Read the model definition and answer for the solid it produces. Units are mm, in the model's axes. A direction names the side the tool comes from. Coordinates: 2 decimals unless noted, no trailing zeros. Write each loop counter-clockwise with the first axis right and the second up, starting at its lowest first coordinate (ties: lowest second). Pieces come first, ordered by that corner, then holes. Notation, with made-up numbers: (-27.75, -36) -> (25.25, -36) arc R31 ccw to (25.25, 1) -> close; hole circle Ø4 at (2, -20.5). An arc over 180 degrees is marked (long way). Return JSON: item names as keys, results as strings.
from build123d import *

# Parameters (mm, degrees)
F1_DEPTH = 50
F3_DEPTH = 50.001


with BuildPart() as f1:
    # F0 (on Front) → F1 (new body)
    with BuildSketch(Plane.XZ):
        Polygon((52.302633, -25), (52.302633, 25), (-47.697367, 25), (-77.697367, -25), (-47.697367, -25), (27.302633, -25), align=None)
        with BuildLine():
            ThreePointArc((-47.697367, -18.25), (-48.581251, -16.116117), (-46.447367, -17))
            ThreePointArc((-46.447367, -17), (-46.813484, -17.883883), (-47.697367, -18.25))
        make_face(mode=Mode.SUBTRACT)
        with BuildLine():
            ThreePointArc((27.302633, -18.25), (26.418749, -16.116117), (28.552633, -17))
            ThreePointArc((28.552633, -17), (28.186516, -17.883883), (27.302633, -18.25))
        make_face(mode=Mode.SUBTRACT)
    extrude(amount=F1_DEPTH)

    # F2 (on face) → F3 (cut, through all)
    with BuildSketch(Plane.XZ.offset(50)):
        Polygon((-47.697367, 25), (-62.697367, 0), (-28.942954, 0), (7.452939, 0), (52.302633, 15.462308), (52.302633, 25), align=None)
    extrude(amount=-F3_DEPTH, mode=Mode.SUBTRACT)


solid = f1.part
1. A tool of negligible diameter and unlimited length cuts with its end or side. For faces 4 (the face through (52.303, -25, -5)), 5 (the face through (-28, -25, 0)), from which of +Z, -Z, +X, -X, +Y, -Y can it reach the whole face along a straight path? Write none if from no direction.
Taken from the geometry:
{"face 4": "+Z, -Z, +X, +Y, -Y", "face 5": "+Z, -X, +Y, -Y"}
2. The part is cut by section A-A (y = -31.5). Determine the outline of the cut face in (x, z).
Taken from the geometry:
{"outline": "(-77.7, -25) -> (52.3, -25) -> (52.3, 15.46) -> (7.45, 0) -> (-62.7, 0) -> close; hole (-47.7, -18.25) arc R1.25 ccw to (-46.45, -17) arc R1.25 ccw (long way) to start; hole (27.3, -18.25) arc R1.25 ccw to (28.55, -17) arc R1.25 ccw (long way) to start"}
3. The part is cut by section B-B (x = -17). Determine the outline of the cut face in (y, z), then the cut area to 3 significant figures.
Taken from the geometry:
{"outline": "(-50, -25) -> (0, -25) -> (0, 0) -> (-50, 0) -> close", "area": "1,250 mm2"}
4. For a pull along Z with two mould halves and no side action, classify faces 1 (the face through (29.56, -25.35, 7.62)), 2 (the face through (-14, -25, -25)), 3 (the face through (1, 0, -13)) as +Z half, -Z half, draft (parallel to the pull), parting line (faces both ways), or undercut.
Taken from the geometry:
{"face 1": "+Z half", "face 2": "-Z half", "face 3": "draft"}
5. The part is cut by section C-C (z = 9). Determine the outline of the cut face in (x, y).
Taken from the geometry:
{"outline": "(33.56, -50) -> (52.3, -50) -> (52.3, 0) -> (33.56, 0) -> close"}
6. Consider L1, parallel to X at y = -43.5, z = -16; L2, parallel to X at y = -29.5, z = -17; L3, parallel to Z at x = -28.5, y = -21. Determine where each line is inside the solid, lowest interval first.
Taken from the geometry:
{"L1": "x = -72.3 to -48.45, -46.95 to 26.55, 28.05 to 52.3", "L2": "x = -72.9 to -48.95, -46.45 to 26.05, 28.55 to 52.3", "L3": "z = -25 to 0"}
7. Flat-ended cylindrical pins translate along their axes: pin 1 Ø8 at (x, y) = (-4, -31.5) entering from +Z; pin 2 Ø1 at (y, z) = (-22.5, -2.5) entering from -X. Find the tip coordinate at first contact, or state that the pin passes through.
Taken from the geometry:
{"pin 1": "stops at z = 0", "pin 2": "stops at x = -64.5"}
